Could you check a few things on this model? Use its own coordinates, in mm. Face numbers are marked on the shaded views. A direction names the side the tool comes from. Give positions to 0.01 mm unless a question says otherwise; leave off trailing zeros. Loops run counter-clockwise (first coordinate to the right, second up) from the corner with the lowest first, then second, coordinate; pieces in that order, holes last. Notation, with made-up numbers: (79, 8) - (85, 8) arc R20 ccw to (85, 23) - close; hole circle Ø9 at (81.5, 80.25). An arc over 180 degrees is marked (long way). Use CSV: the item, a comma, the result in double quotes.
from build123d import *

# Parameters (mm, degrees)
BOSS_EXTRUDE1_DEPTH     = 0.9
SKETCH8_R               = 3
SKETCH8_R_2             = 2.5
BOSS_EXTRUDE2_DEPTH     = 1.2
SKETCH1_R               = 2.5
CUT_EXTRUDE1_DEPTH      = 11.070253224
CUT_EXTRUDE1_DEPTH_BACK = 11.070253224


with BuildPart() as part:
    # Sketch7 → Boss-Extrude1 (new, symmetric)
    with BuildSketch(Plane.XY):
        with BuildLine():
            Line((-7.92820323, 4), (4.92820323, 4))
            ThreePointArc((4.92820323, 4), (6, 0), (4.92820323, -4))
            Line((4.92820323, -4), (-7.92820323, -4))
            ThreePointArc((-7.92820323, -4), (-9, 0), (-7.92820323, 4))
        make_face()
    extrude(amount=BOSS_EXTRUDE1_DEPTH, both=True)

    # Sketch8 → Boss-Extrude2 (add)
    with BuildSketch(Plane.XY.offset(0.9)):
        with Locations(Location((0, 0, 0), (0, 0, 180))):
            Circle(SKETCH8_R)
        Circle(SKETCH8_R_2, mode=Mode.SUBTRACT)
    extrude(amount=BOSS_EXTRUDE2_DEPTH)

    # Sketch1 → Cut-Extrude1 (cut, two sides)
    with BuildSketch(Plane.XY) as cut_extrude1_sk:
        Circle(SKETCH1_R)
    extrude(amount=CUT_EXTRUDE1_DEPTH, mode=Mode.SUBTRACT)
    extrude(cut_extrude1_sk.sketch, amount=-CUT_EXTRUDE1_DEPTH_BACK, mode=Mode.SUBTRACT)


solid = part.part
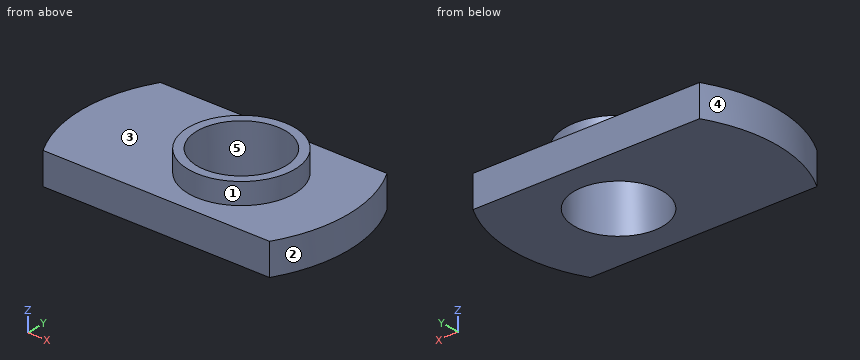
1) Which directions (+Z, -Z, +X, -X, +Y, -Y) give clear straight access to the entire face, cutting with the end or side of a thin tool? Please do the marked faces 1 and 2.
Answer below:
face 1,"+Z"
face 2,"+Z, -Z, +X"
2) I'm going to push flat-ended pins straight in: P1, Ø1.5, axis at y = -2.5, z = -0.5, coming from the +X side; P2, Ø4, axis at x = 0, y = 0, coming from the -Z side; P3, Ø1, axis at x = 3, z = 1.5, coming from the +Y side. Where does each tip first touch, or does it pass through?
Answer below:
P1,"stops at x = 5.81"
P2,"passes through"
P3,"stops at y = 1.66"
3) We'd pull the mould along Y, two halves only. Please class the marked faces 3, 4 and 5: +Y half, -Y half, draft (parallel to the pull), parting line (faces both ways), or undercut.
Answer below:
face 3,"draft"
face 4,"parting line"
face 5,"undercut"
4) Suppose I cut it at A-A (y = 0). Please give me the cut outline in (x, z).
Answer below:
outline,"(-9, -0.9) - (-2.5, -0.9) - (-2.5, 2.1) - (-3, 2.1) - (-3, 0.9) - (-9, 0.9) - close; (2.5, -0.9) - (6, -0.9) - (6, 0.9) - (3, 0.9) - (3, 2.1) - (2.5, 2.1) - close"
5) Suppose I cut it at D-D (x = -6.75). Please give me the cut outline in (y, z).
Answer below:
outline,"(-4, -0.9) - (4, -0.9) - (4, 0.9) - (-4, 0.9) - close"
6) Suppose I cut it at B-B (x = 0). Please give me the cut outline in (y, z).
Answer below:
outline,"(-4, -0.9) - (-2.5, -0.9) - (-2.5, 2.1) - (-3, 2.1) - (-3, 0.9) - (-4, 0.9) - close; (2.5, -0.9) - (4, -0.9) - (4, 0.9) - (3, 0.9) - (3, 2.1) - (2.5, 2.1) - close"
7) I need wall thicknesses on line 1 along Y through (x, z) = (0, 0.1); line 2 along Y through (x, z) = (0, 1.15); line 3 along Z through (x, y) = (-6.5, -1.5). Which ranges of each line are inside material? Lowest first, please.
Answer below:
line 1,"y = -4 to -2.5, 2.5 to 4"
line 2,"y = -3 to -2.5, 2.5 to 3"
line 3,"z = -0.9 to 0.9"
8) Suppose I cut it at C-C (z = 0.1). Please give me the cut outline in (x, y), plus the area to 3 significant figures.
Answer below:
outline,"(-7.93, -4) - (4.93, -4) arc R8 ccw to (4.93, 4) - (-7.93, 4) arc R8 ccw to start; hole circle Ø5 at (0, 0)"
area,"94.8 mm2"
